Geometry check sheet. Reference: the model listing, model coordinates, mm. Give positions to 0.01 mm unless a question says otherwise; leave off trailing zeros. Loops run counter-clockwise (first coordinate to the right, second up) from the corner with the lowest first, then second, coordinate; pieces in that order, holes last.
```python
from build123d import *

# Parameters (mm, degrees)
F0_W     = 266.7
F0_H     = 152.4
F0_R     = 19.05
F1_DEPTH = 50.8
F2_R     = 6.35


with BuildPart() as f1:
    # F0 (on Front) → F1 (new body)
    with BuildSketch(Plane.XZ):
        Rectangle(F0_W, F0_H)
        with Locations((-63.2546767592, 0)):
            Circle(F0_R, mode=Mode.SUBTRACT)
        with BuildLine():
            ThreePointArc((-19.05, 0), (0, 19.05), (19.05, 0))
            ThreePointArc((19.05, 0), (0, -19.05), (-19.05, 0))
        make_face(mode=Mode.SUBTRACT)
        with Locations((63.8258159161, 0)):
            Circle(F0_R, mode=Mode.SUBTRACT)
    extrude(amount=F1_DEPTH)

    # F2
    f2_edges = [f1.edges().sort_by_distance(p)[0] for p in [
        (0, -50.8, -76.2),
        (133.35, -50.8, 0),
        (0, -50.8, 76.2),
        (-133.35, -50.8, 0),
        (0, 0, 76.2),
        (133.35, 0, 0),
        (0, 0, -76.2),
        (-133.35, 0, 0),
    ]]
    fillet(f2_edges, radius=F2_R)


solid = f1.part
```
1) Sectioned sample at A-A on z = 0. Enter the section's corners in (x, y), plus the area to 3 significant figures.
2) Sectioned sample at C-C on y = -9.5. Enter the section's corners in (x, z), plus the area to 3 significant figures.
3) Sectioned sample at D-D on x = -56. Enter the section's corners in (y, z).
4) Scan lines: line 1 along Z through (x, y) = (0, -24); line 2 along X through (y, z) = (-39, 13); line 3 along Y through (x, z) = (75.5, 70). Record each from-to range of solid material in increasing order.
5) Mould release check, pull along Z, two halves, no side actions. Record for faces 1 (the cylindrical face through (-45.084, -25.044, 5.722)), 2 (the cylindrical face through (1.87, -1.91, 74.39)), 3 (the flat face through (26, -50.8, 1)), 4 (the flat face through (-2, -25, -76.2)): +Z half, -Z half, draft (parallel to the pull), parting line (faces both ways), or undercut.
6) Sectioned sample at B-B on x = 0. Enter the section's corners in (y, z).
Determined:
1. outline: (-133.35, -44.45) arc R6.35 ccw to (-127, -50.8) - (-82.3, -50.8) - (-82.3, 0) - (-127, 0) arc R6.35 ccw to (-133.35, -6.35) - close; (-44.2, -50.8) - (-19.05, -50.8) - (-19.05, 0) - (-44.2, 0) - close; (19.05, -50.8) - (44.78, -50.8) - (44.78, 0) - (19.05, 0) - close; (82.88, -50.8) - (127, -50.8) arc R6.35 ccw to (133.35, -44.45) - (133.35, -6.35) arc R6.35 ccw to (127, 0) - (82.88, 0) - close
1. area: 7,710 mm2
2. outline: (-133.35, -76.2) - (133.35, -76.2) - (133.35, 76.2) - (-133.35, 76.2) - close; hole circle Ø38.1 at (-63.25, 0); hole circle Ø38.1 at (0, 0); hole circle Ø38.1 at (63.83, 0)
2. area: 37,200 mm2
3. outline: (-50.8, -69.85) arc R6.35 ccw to (-44.45, -76.2) - (-6.35, -76.2) arc R6.35 ccw to (0, -69.85) - (0, -17.61) - (-50.8, -17.61) - close; (-50.8, 17.61) - (0, 17.61) - (0, 69.85) arc R6.35 ccw to (-6.35, 76.2) - (-44.45, 76.2) arc R6.35 ccw to (-50.8, 69.85) - close
4. line 1: z = -76.2 to -19.05, 19.05 to 76.2
4. line 2: x = -133.35 to -77.18, -49.33 to -13.92, 13.92 to 49.9, 77.75 to 133.35
4. line 3: y = -50.8 to 0
5. face 1: undercut
5. face 2: +Z half
5. face 3: draft
5. face 4: -Z half
6. outline: (-50.8, -69.85) arc R6.35 ccw to (-44.45, -76.2) - (-6.35, -76.2) arc R6.35 ccw to (0, -69.85) - (0, -19.05) - (-50.8, -19.05) - close; (-50.8, 19.05) - (0, 19.05) - (0, 69.85) arc R6.35 ccw to (-6.35, 76.2) - (-44.45, 76.2) arc R6.35 ccw to (-50.8, 69.85) - close
